from build123d import *

# Parameters (mm, degrees)
SKETCH1_R           = 88.9
BOSS_EXTRUDE1_DEPTH = 40
SKETCH2_R           = 82.55
BOSS_EXTRUDE2_DEPTH = 10
SKETCH3_W           = 30
SKETCH3_H           = 35
CUT_EXTRUDE1_DEPTH  = 5


with BuildPart() as part:
    # Sketch1 → Boss-Extrude1 (new body)
    with BuildSketch(Plane(origin=(0, 0, 0), x_dir=(1, 0, 0), z_dir=(0, 1, 0))):
        with Locations(Location((0, 0, 0), (0, 0, 270))):
            Circle(SKETCH1_R)
    extrude(amount=BOSS_EXTRUDE1_DEPTH)

    # Sketch2 → Boss-Extrude2 (add)
    with BuildSketch(Plane(origin=(0, 40, 0), x_dir=(1, 0, 0), z_dir=(0, 1, 0))):
        with Locations(Location((0, 0, 0), (0, 0, 270))):
            Circle(SKETCH2_R)
    extrude(amount=BOSS_EXTRUDE2_DEPTH)

    # Sketch3 → Cut-Extrude1 (cut, symmetric)
    with BuildSketch(Plane.XY):
        with Locations((0, 32.5)):
            Rectangle(SKETCH3_W, SKETCH3_H)
    extrude(amount=CUT_EXTRUDE1_DEPTH, both=True, mode=Mode.SUBTRACT)


solid = part.part
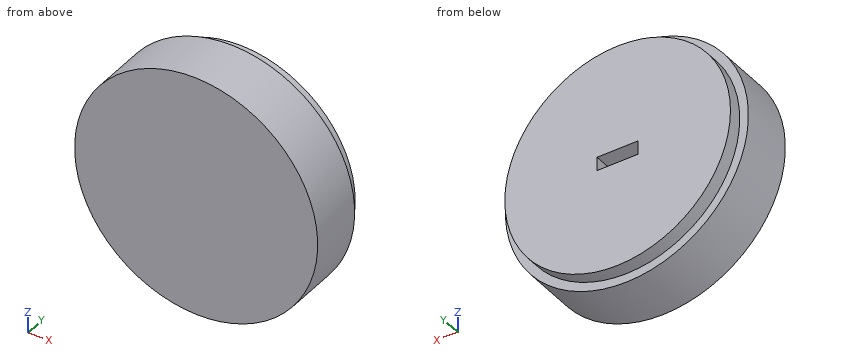
Could you check a few things on this model? Use its own coordinates, in mm. Coordinates: 2 decimals unless noted, no trailing zeros. Order: outer loops, then holes, each group sorted by start corner. A loop starts at its lowest first (then second) coordinate and runs counter-clockwise, first axis right, second up. Notation, with made-up numbers: (46.25, -35.5) - (60.25, -35.5) arc R30 ccw to (60.25, 1.5) - close; hole circle Ø7 at (35, 56.25). An arc over 180 degrees is marked (long way). Answer in a Markdown table with one row per item. Add a question column.
(1) If we section it at B-B, the plane y = 21.5: Please give me the cut outline in (x, z), then the cut area to 3 significant figures.
(2) If we section it at A-A, the plane x = 0: Please give me the cut outline in (y, z).
(3) If we section it at D-D, the plane y = 9.5: Please give me the cut outline in (x, z).
(4) I need wall thicknesses on L1, parallel to Y at x = -67, z = -57; L2, parallel to Z at x = -13, y = 33.5; L3, parallel to Z at x = -4.5, y = 24. Which ranges of each line are inside material? Lowest first, please.
(5) If we section it at C-C, the plane z = -19.5: Please give me the cut outline in (x, y) (3 decimals), then the cut area to 3 significant figures.
(6) Will these pins go through, and if not, where does the flat tip stop? pin 1 (3 mm diameter, centred on x = -4.5, z = 1.5, fed in from +Y); pin 2 (2 mm diameter, centred on x = 53, y = 6.5, fed in from -Z); pin 3 (5 mm diameter, centred on y = 20, z = 35.5, fed in from +X); pin 4 (5 mm diameter, centred on x = 59.5, z = 34, fed in from -Y).
Results are:
| question | item | result |
|---|---|---|
| 1 | outline | circle Ø177.8 at (0, 0); hole (-15, -5) - (15, -5) - (15, 5) - (-15, 5) - close |
| 1 | area | 24,500 mm2 |
| 2 | outline | (0, -88.9) - (40, -88.9) - (40, -82.55) - (50, -82.55) - (50, -5) - (15, -5) - (15, 5) - (50, 5) - (50, 82.55) - (40, 82.55) - (40, 88.9) - (0, 88.9) - close |
| 3 | outline | circle Ø177.8 at (0, 0) |
| 4 | L1 | y = 0 to 40 |
| 4 | L2 | z = -87.94 to -5, 5 to 87.94 |
| 4 | L3 | z = -88.79 to -5, 5 to 88.79 |
| 5 | outline | (-86.735, 0) - (86.735, 0) - (86.735, 40) - (80.214, 40) - (80.214, 50) - (-80.214, 50) - (-80.214, 40) - (-86.735, 40) - close |
| 5 | area | 8,540 mm2 |
| 6 | pin 1 | stops at y = 15 |
| 6 | pin 2 | stops at z = -72.11 |
| 6 | pin 3 | stops at x = 82.55 |
| 6 | pin 4 | stops at y = 0 |
